```python
from build123d import *

# Parameters (mm, degrees)
F1_DEPTH = 50.8


with BuildPart() as f1:
    # F0 (on Front) → F1 (new body)
    with BuildSketch(Plane.XZ):
        with BuildLine():
            ThreePointArc((0, 35.790812), (-25.307926, 25.307926), (-35.790812, 0))
            Line((-35.790812, 0), (0, 0))
            Line((0, 0), (0, 35.790812))
        make_face()
        Polygon((0, 0), (-35.790812, 0), (-35.877675, 0), (-35.877675, -58.146574), (0, -58.146574), align=None)
    extrude(amount=F1_DEPTH)


solid = f1.part
```
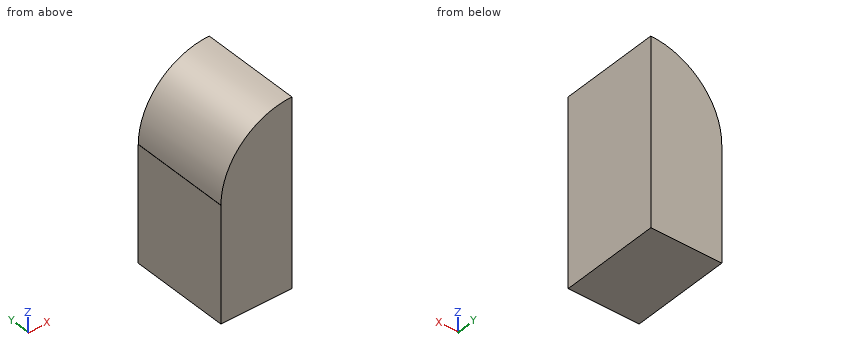
Verification items for the finished model (mm, model axes). Round coordinates to 2 decimals unless told otherwise and drop trailing zeros. Write each loop counter-clockwise with the first axis right and the second up, starting at its lowest first coordinate (ties: lowest second). Pieces come first, ordered by that corner, then holes. Notation, with made-up numbers: (76.25, 4) -> (130.25, 4) arc R22 ccw to (130.25, 42) -> close; hole circle Ø10 at (73, 81). An arc over 180 degrees is marked (long way). Write each question's results on one line, items separated by ' | '. Start each with the question number.
1. Cross-section at A-A (y = -23.5). Enter the section's corners in (x, z), then the cut area to 3 significant figures.
2. Material ranges on probe 1 along Z at (x, y) = (-21, -24); probe 2 along Z at (x, y) = (-15, -23.5); probe 3 along X at (y, z) = (-11.5, 14), recorded low to high. Write a range as from..to.
3. Cross-section at C-C (z = 18.5). Enter the section's corners in (x, y).
4. Cross-section at B-B (x = -29). Enter the section's corners in (y, z), then the cut area to 3 significant figures.
Solutions:
1) outline: (-35.88, -58.15) -> (0, -58.15) -> (0, 35.79) arc R35.79 ccw to (-35.79, 0) -> (-35.88, 0) -> close | area: 3,090 mm2
2) probe 1: z = -58.15..28.98 | probe 2: z = -58.15..32.5 | probe 3: x = -32.94..0
3) outline: (-30.64, -50.8) -> (0, -50.8) -> (0, 0) -> (-30.64, 0) -> close
4) outline: (-50.8, -58.15) -> (0, -58.15) -> (0, 20.98) -> (-50.8, 20.98) -> close | area: 4,020 mm2
